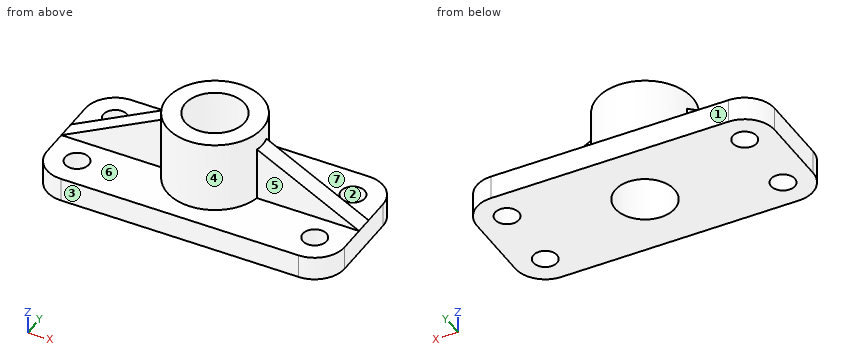
```python
from build123d import *

# Parameters (mm, degrees)
F0_R     = 6.35
F1_DEPTH = 12.7
F2_R     = 25.4
F3_DEPTH = 38.1
F5_DEPTH = 4.7625
F6_R     = 15.875
F7_DEPTH = 50.801


with BuildPart() as f1:
    # F0 (on Top) → F1 (new body)
    with BuildSketch(Plane.XY):
        with BuildLine():
            Line((-63.5, -35.076942), (0, -35.076942))
            Line((0, -35.076942), (63.5, -35.076942))
            ThreePointArc((63.5, -35.076942), (74.83276, -30.38276), (79.526942, -19.05))
            Line((79.526942, -19.05), (79.526942, 0))
            Line((79.526942, 0), (79.526942, 19.05))
            ThreePointArc((79.526942, 19.05), (74.83276, 30.38276), (63.5, 35.076942))
            Line((63.5, 35.076942), (0, 35.076942))
            Line((0, 35.076942), (-63.5, 35.076942))
            ThreePointArc((-63.5, 35.076942), (-74.83276, 30.38276), (-79.526942, 19.05))
            Line((-79.526942, 19.05), (-79.526942, 0))
            Line((-79.526942, 0), (-79.526942, -19.05))
            ThreePointArc((-79.526942, -19.05), (-74.83276, -30.38276), (-63.5, -35.076942))
        make_face()
        with Locations((-63.5, -19.05)):
            Circle(F0_R, mode=Mode.SUBTRACT)
        with Locations((63.5, -19.05)):
            Circle(F0_R, mode=Mode.SUBTRACT)
        with Locations((-63.5, 19.05)):
            Circle(F0_R, mode=Mode.SUBTRACT)
        with Locations((63.5, 19.05)):
            Circle(F0_R, mode=Mode.SUBTRACT)
    extrude(amount=-F1_DEPTH)

    # F2 (on face) → F3 (join)
    with BuildSketch(Plane.XY):
        Circle(F2_R)
    extrude(amount=F3_DEPTH)

    # F4 (on Front) → F5 (join, symmetric)
    with BuildSketch(Plane.XZ):
        Polygon((-19.05, 31.75), (-79.5274, 0), (79.5274, 0), (19.05, 31.75), align=None)
    extrude(amount=F5_DEPTH, both=True)

    # F6 (on face) → F7 (cut, through all)
    with BuildSketch(Plane.XY.offset(38.1)):
        Circle(F6_R)
    extrude(amount=-F7_DEPTH, mode=Mode.SUBTRACT)


solid = f1.part
```
Work out the finished part from the listing and answer in its coordinate system (mm). Face numbers are marked on the shaded views. A direction names the side the tool comes from. Coordinates: 2 decimals unless noted, no trailing zeros. Write each loop counter-clockwise with the first axis right and the second up, starting at its lowest first coordinate (ties: lowest second). Pieces come first, ordered by that corner, then holes.
Q1. Each of these flat-tipped pins is pushed along its axis until it touches: pin 1 Ø10 at (x, z) = (-9.5, 32.5) entering from +Y; pin 2 Ø3 at (y, z) = (-25, 21.5) entering from -X; pin 3 Ø20.5 at (x, y) = (-63.5, -19.05) entering from +Z; pin 4 Ø10 at (x, y) = (63.5, -19.05) entering from -Z. Where does it stop, or does it pass through?
Q2. A cutting plane is placed at A-A, the plane x = 0. Give the vertices of the cut face in (y, z) (3 decimals).
Q3. A cutting plane is placed at B-B, the plane z = -2. Give the vertices of the cut face in (x, y) (3 decimals), then the cut area to 3 significant figures.
Q4. Which of the six approach directions +Z, -Z, +X, -X, +Y, -Y give full straight-line access (tool end or side, diameter ignored) to the marked faces 4, 5, 6 and 7?
Q5. Determine the mould class of the marked faces 1, 2 and 3 for opening direction Y: released by +Y, released by -Y, zero draft, split by the parting line, or undercut.
Q6. Find the intervals of material crossed by line 1 (Y direction, x = 63, z = -4); line 2 (X direction, y = 19, z = -4); line 3 (Z direction, x = 69, y = -31), in increasing order.
Q7. A cutting plane is placed at D-D, the plane y = 22.5. Give the vertices of the cut face in (x, z).
Findings below:
1. pin 1: stops at y = 25
1. pin 2: stops at x = -9.64
1. pin 3: stops at z = 0
1. pin 4: passes through
2. outline: (-35.077, -12.7) - (-15.875, -12.7) - (-15.875, 38.1) - (-25.4, 38.1) - (-25.4, 0) - (-35.077, 0) - close; (15.875, -12.7) - (35.077, -12.7) - (35.077, 0) - (25.4, 0) - (25.4, 38.1) - (15.875, 38.1) - close
3. outline: (-79.527, -19.05) arc R16.027 ccw to (-63.5, -35.077) - (63.5, -35.077) arc R16.027 ccw to (79.527, -19.05) - (79.527, 19.05) arc R16.027 ccw to (63.5, 35.077) - (-63.5, 35.077) arc R16.027 ccw to (-79.527, 19.05) - close; hole circle Ø12.7 at (-63.5, -19.05); hole circle Ø12.7 at (-63.5, 19.05); hole circle Ø31.75 at (0, 0); hole circle Ø12.7 at (63.5, -19.05); hole circle Ø12.7 at (63.5, 19.05)
3. area: 9,640 mm2
4. face 4: +Z
4. face 5: +Z, +X, -Y
4. face 6: +Z, -Y
4. face 7: +Z, +Y
5. face 1: released by +Y
5. face 2: undercut
5. face 3: released by -Y
6. line 1: y = -35.08 to -25.38, -12.72 to 12.72, 25.38 to 35.08
6. line 2: x = -79.53 to -69.85, -57.15 to 57.15, 69.85 to 79.53
6. line 3: z = -12.7 to 0
7. outline: (-79.15, -12.7) - (-68.83, -12.7) - (-68.83, 0) - (-79.15, 0) - close; (-58.17, -12.7) - (58.17, -12.7) - (58.17, 0) - (11.79, 0) - (11.79, 38.1) - (-11.79, 38.1) - (-11.79, 0) - (-58.17, 0) - close; (68.83, -12.7) - (79.15, -12.7) - (79.15, 0) - (68.83, 0) - close
